```python
from build123d import *

# Parameters (mm, degrees)
SKETCH_1_R          = 178
EXTRUDE_1_DEPTH     = 4
SKETCH_2_R          = 10.414
SKETCH_2_R_2        = 5.2
CUT_EXTRUDE_1_DEPTH = 10
SKETCH_4_R          = 54.5
CUT_EXTRUDE_2_DEPTH = 10
SKETCH_5_R          = 2
CUT_EXTRUDE_3_DEPTH = 10
CUT_EXTRUDE_4_DEPTH = 10
SKETCH_11_W         = 100
SKETCH_11_H         = 3
CUT_EXTRUDE_5_DEPTH = 10
SKETCH_13_R         = 15
CUT_EXTRUDE_6_DEPTH = 10


with BuildPart() as part:
    # 草图1 → 凸台-拉伸1 (new body)
    with BuildSketch(Plane(origin=(0, 0, 0), x_dir=(1, 0, 0), z_dir=(0, 1, 0))):
        Circle(SKETCH_1_R)
    extrude(amount=EXTRUDE_1_DEPTH)

    # 草图2 → 切除-拉伸1 (cut)
    with BuildSketch(Plane(origin=(0, 4, 0), x_dir=(1, 0, 0), z_dir=(0, 1, 0))):
        with Locations((115.258405333, 115.258405333)):
            Circle(SKETCH_2_R)
        with Locations((-90.216925784, -106.480381752)):
            Circle(SKETCH_2_R_2)
        with Locations((-106.480381752, -90.216925784)):
            Circle(SKETCH_2_R_2)
        with Locations((115.258405333, -115.258405333)):
            Circle(SKETCH_2_R)
        with Locations((-115.258405333, -115.258405333)):
            Circle(SKETCH_2_R)
        with Locations((-115.258405333, 115.258405333)):
            Circle(SKETCH_2_R)
        with Locations((-90.216925784, 106.480381752)):
            Circle(SKETCH_2_R_2)
        with Locations((-106.480381752, 90.216925784)):
            Circle(SKETCH_2_R_2)
        with Locations((106.480381752, 90.216925784)):
            Circle(SKETCH_2_R_2)
        with Locations((90.216925784, 106.480381752)):
            Circle(SKETCH_2_R_2)
        with Locations((90.216925784, -106.480381752)):
            Circle(SKETCH_2_R_2)
        with Locations((106.480381752, -90.216925784)):
            Circle(SKETCH_2_R_2)
    extrude(amount=-CUT_EXTRUDE_1_DEPTH, mode=Mode.SUBTRACT)

    # 草图4 → 切除-拉伸2 (cut)
    with BuildSketch(Plane.XZ):
        with Locations((80.5, 0)):
            Circle(SKETCH_4_R)
        with Locations((-80.5, 0)):
            Circle(SKETCH_4_R)
    extrude(amount=-CUT_EXTRUDE_2_DEPTH, mode=Mode.SUBTRACT)

    # 草图5 → 切除-拉伸3 (cut)
    with BuildSketch(Plane(origin=(0, 4, 0), x_dir=(1, 0, 0), z_dir=(0, 1, 0))):
        with Locations((-19.5, -14.8)):
            Circle(SKETCH_5_R)
        with Locations((-4.5, -14.8)):
            Circle(SKETCH_5_R)
        with Locations((-4.5, 14.8)):
            Circle(SKETCH_5_R)
        with Locations((-19.5, 14.8)):
            Circle(SKETCH_5_R)
        with Locations((4.5, -14.8)):
            Circle(SKETCH_5_R)
        with Locations((19.5, -14.8)):
            Circle(SKETCH_5_R)
        with Locations((19.5, 14.8)):
            Circle(SKETCH_5_R)
        with Locations((4.5, 14.8)):
            Circle(SKETCH_5_R)
        with Locations((-65.7, -61)):
            Circle(SKETCH_5_R)
        with Locations((-65.7, -76)):
            Circle(SKETCH_5_R)
        with Locations((-95.3, -61)):
            Circle(SKETCH_5_R)
        with Locations((-95.3, -76)):
            Circle(SKETCH_5_R)
        with Locations((-141.5, -14.8)):
            Circle(SKETCH_5_R)
        with Locations((-156.5, -14.8)):
            Circle(SKETCH_5_R)
        with Locations((-141.5, 14.8)):
            Circle(SKETCH_5_R)
        with Locations((-156.5, 14.8)):
            Circle(SKETCH_5_R)
        with Locations((-95.3, 61)):
            Circle(SKETCH_5_R)
        with Locations((-95.3, 76)):
            Circle(SKETCH_5_R)
        with Locations((-65.7, 61)):
            Circle(SKETCH_5_R)
        with Locations((-65.7, 76)):
            Circle(SKETCH_5_R)
        with Locations((95.3, 76)):
            Circle(SKETCH_5_R)
        with Locations((95.3, 61)):
            Circle(SKETCH_5_R)
        with Locations((65.7, 76)):
            Circle(SKETCH_5_R)
        with Locations((65.7, 61)):
            Circle(SKETCH_5_R)
        with Locations((156.5, -14.8)):
            Circle(SKETCH_5_R)
        with Locations((141.5, -14.8)):
            Circle(SKETCH_5_R)
        with Locations((156.5, 14.8)):
            Circle(SKETCH_5_R)
        with Locations((141.5, 14.8)):
            Circle(SKETCH_5_R)
        with Locations((65.7, -76)):
            Circle(SKETCH_5_R)
        with Locations((65.7, -61)):
            Circle(SKETCH_5_R)
        with Locations((95.3, -76)):
            Circle(SKETCH_5_R)
        with Locations((95.3, -61)):
            Circle(SKETCH_5_R)
    extrude(amount=-CUT_EXTRUDE_3_DEPTH, mode=Mode.SUBTRACT)

    # 草图8 → 切除-拉伸4 (cut)
    with BuildSketch(Plane.XZ):
        with BuildLine():
            Line((95.833188406, 150), (0, 150))
            Line((0, 150), (-95.833188406, 150))
            ThreePointArc((-95.833188406, 150), (0, 178), (95.833188406, 150))
        make_face()
        with BuildLine():
            Line((170, 52.763623833), (170, 0))
            Line((170, 0), (170, -52.763623833))
            ThreePointArc((170, -52.763623833), (178, 0), (170, 52.763623833))
        make_face()
        with BuildLine():
            Line((0, -150), (-95.833188406, -150))
            ThreePointArc((-95.833188406, -150), (0, -178), (95.833188406, -150))
            Line((95.833188406, -150), (0, -150))
        make_face()
        with BuildLine():
            Line((-170, 0), (-170, -52.763623833))
            ThreePointArc((-170, -52.763623833), (-178, 0), (-170, 52.763623833))
            Line((-170, 52.763623833), (-170, 0))
        make_face()
    extrude(amount=-CUT_EXTRUDE_4_DEPTH, mode=Mode.SUBTRACT)

    # 草图11 → 切除-拉伸5 (cut)
    with BuildSketch(Plane.XZ):
        with Locations((0, -86.5)):
            Rectangle(SKETCH_11_W, SKETCH_11_H)
        Polygon((65, -135), (30, -135), (30, -119), (30, -103), (65, -103), align=None)
        Polygon((-65, -119), (-65, -103), (-30, -103), (-30, -119), (-30, -135), (-65, -135), align=None)
        with Locations((0, 86.5)):
            Rectangle(SKETCH_11_W, SKETCH_11_H)
        Polygon((-65, 119), (-65, 103), (-30, 103), (-30, 119), (-30, 135), (-65, 135), align=None)
        Polygon((65, 103), (65, 135), (30, 135), (30, 119), (30, 103), align=None)
    extrude(amount=-CUT_EXTRUDE_5_DEPTH, mode=Mode.SUBTRACT)

    # 草图13 → 切除-拉伸6 (cut)
    with BuildSketch(Plane.XZ):
        with Locations((0, -50)):
            Circle(SKETCH_13_R)
        with Locations((0, 50)):
            Circle(SKETCH_13_R)
    extrude(amount=-CUT_EXTRUDE_6_DEPTH, mode=Mode.SUBTRACT)


solid = part.part
```
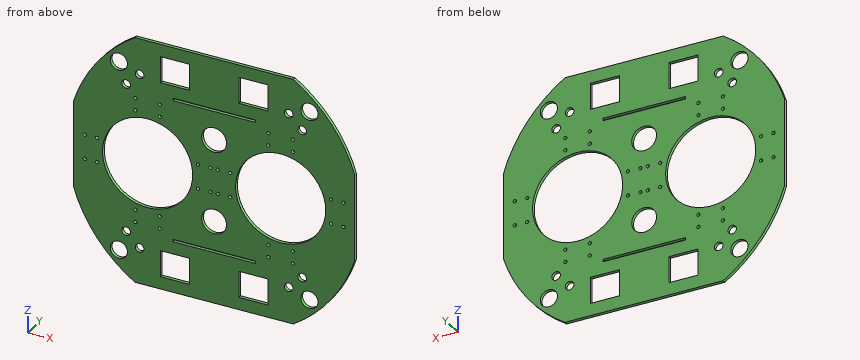
Read the model definition and answer for the solid it produces. Units are mm, in the model's axes. Give positions to 0.01 mm unless a question says otherwise; leave off trailing zeros. Loops run counter-clockwise (first coordinate to the right, second up) from the corner with the lowest first, then second, coordinate; pieces in that order, holes last.
Item 1: Find the intervals of material crossed by line 1 along Z through (x, y) = (-79, 3.4); line 2 along X through (y, z) = (2.15, 76); line 3 along Z through (x, y) = (48, 2.6), in increasing order.
Item 2: Each of these flat-tipped pins is pushed along its axis until it touches: pin 1 Ø2 at (x, z) = (-124.5, 37.5) entering from -Y; pin 2 Ø1 at (x, y) = (111.5, 2) entering from -Z; pin 3 Ø0.9 at (y, z) = (2.5, 86.5) entering from +X; pin 4 Ø3.5 at (x, z) = (-4.5, -14.8) entering from +Y. Where does it stop, or does it pass through?
Item 3: The part is cut by section C-C (x = 121.5). Write down the section's boundary in (y, z), and give its area (3 significant figures).
Item 4: The part is cut by section D-D (y = 3.1). Give the number of separate pieces and of enclosed holes in the cut face, and give its area (3 significant figures).
Item 5: The part is cut by section B-B (z = 45). Write down the section's boundary in (x, y), and give its area (3 significant figures).
Item 6: The part is cut by section A-A (x = -80.5). Write down the section's boundary in (y, z), and give its area (3 significant figures).
Taken from the geometry:
1. line 1: z = -150 to -54.48, 54.48 to 150
1. line 2: x = -160.96 to -97.3, -93.3 to -67.7, -63.7 to 63.7, 67.7 to 93.3, 97.3 to 160.96
1. line 3: z = -150 to -135, -103 to -88, -85 to -43.75, 43.75 to 85, 88 to 103, 135 to 150
2. pin 1: stops at y = 0
2. pin 2: stops at z = -139.15
2. pin 3: stops at x = 155.82
2. pin 4: passes through
3. outline: (0, -130.08) - (4, -130.08) - (4, -123.59) - (0, -123.59) - close; (0, -106.92) - (4, -106.92) - (4, -35.91) - (0, -35.91) - close; (0, 35.91) - (4, 35.91) - (4, 106.92) - (0, 106.92) - close; (0, 123.59) - (4, 123.59) - (4, 130.08) - (0, 130.08) - close
3. area: 620 mm2
4. separate pieces: 1
4. enclosed holes: 54
4. area: 63,500 mm2
5. outline: (-170, 0) - (-111.24, 0) - (-111.24, 4) - (-170, 4) - close; (-49.76, 0) - (-14.14, 0) - (-14.14, 4) - (-49.76, 4) - close; (14.14, 0) - (49.76, 0) - (49.76, 4) - (14.14, 4) - close; (111.24, 0) - (170, 0) - (170, 4) - (111.24, 4) - close
5. area: 755 mm2
6. outline: (0, -150) - (4, -150) - (4, -54.5) - (0, -54.5) - close; (0, 54.5) - (4, 54.5) - (4, 150) - (0, 150) - close
6. area: 764 mm2
